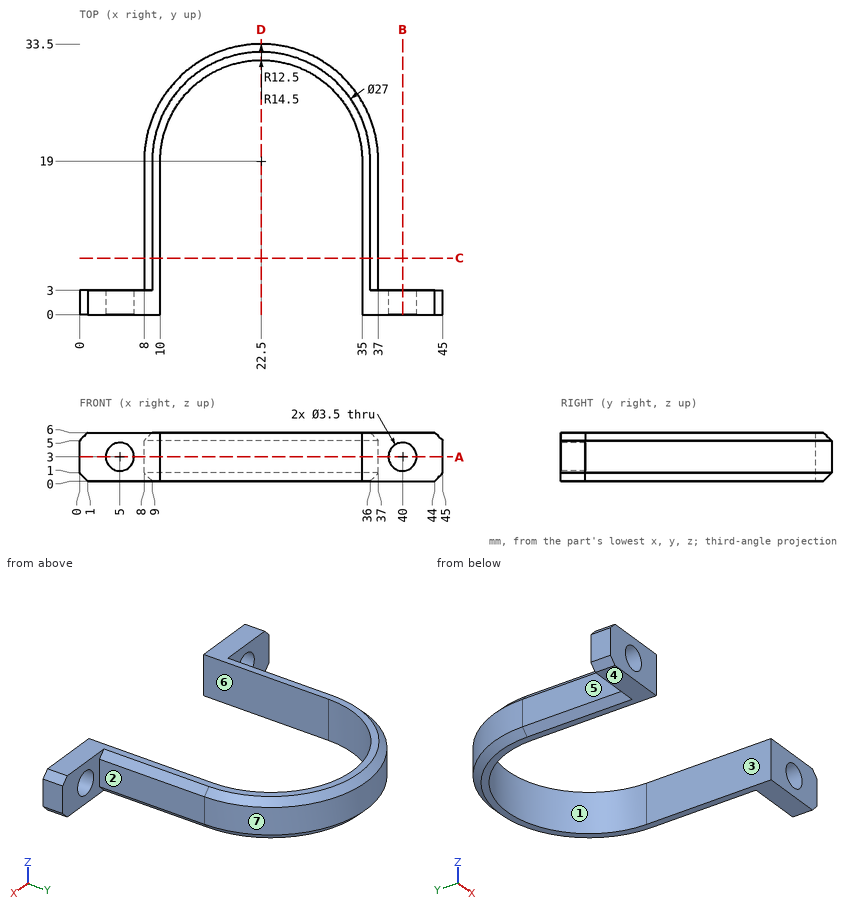
Answer from the drawing. Dimensions are ordinates in mm from the lowest x, y and z of the part. A direction names the side the tool comes from. Round coordinates to 2 decimals unless told otherwise and drop trailing zeros. Loops run counter-clockwise (first coordinate to the right, second up) from the corner with the lowest first, then second, coordinate; pieces in that order, holes last.
1) A cutting plane is placed at D-D on x = 22.5. Determine the outline of the cut face in (y, z).
Outcome:
outline: (31.5, 0) - (32.5, 0) - (33.5, 1) - (33.5, 5) - (32.5, 6) - (31.5, 6) - close
2) Consider line 1 (X direction, y = 16, z = 3.5); line 2 (Z direction, x = 5, y = 1.3); line 3 (X direction, y = 2.5, z = 4). Determine where each line is inside the solid, lowest interval first.
Outcome:
line 1: x = 8 to 10, 35 to 37
line 2: z = 0 to 1.25, 4.75 to 6
line 3: x = 0 to 3.56, 6.44 to 10, 35 to 38.56, 41.44 to 45
3) A cutting plane is placed at B-B on x = 40. Determine the outline of the cut face in (y, z), plus the area to 3 significant figures.
Outcome:
outline: (0, 0) - (3, 0) - (3, 1.25) - (0, 1.25) - close; (0, 4.75) - (3, 4.75) - (3, 6) - (0, 6) - close
area: 7.50 mm2
4) For the marked faces 5, 6 and 7, determine the directions among +Z, -Z, +X, -X, +Y, -Y from which every point of the face is accessible in a straight line to the end or side of a thin tool.
Outcome:
face 5: +Z, -Z, -X, +Y
face 6: +Z, -Z, -Y
face 7: +Z, -Z, +Y
5) A cutting plane is placed at C-C on y = 7. Determine the outline of the cut face in (x, z), plus the area to 3 significant figures.
Outcome:
outline: (8, 1) - (9, 0) - (10, 0) - (10, 6) - (9, 6) - (8, 5) - close; (35, 0) - (36, 0) - (37, 1) - (37, 5) - (36, 6) - (35, 6) - close
area: 22.0 mm2
6) For a pull along X with two mould halves and no side action, classify the marked faces 1, 2, 3 and 4 as released by +X, released by -X, zero draft, split by the parting line, or undercut.
Outcome:
face 1: undercut
face 2: released by +X
face 3: undercut
face 4: zero draft
7) Given P1, Ø2, axis at y = 15.5, z = 4.5, coming from the -X side; P2, Ø2, axis at y = 24.5, z = 4, coming from the +X side; P3, Ø3, axis at y = 8.5, z = 3, coming from the +X side; P4, Ø3, axis at x = 40, z = 3, coming from the -Y side, each flat-ended and moving along its own axis, determine where each tip first touches the part or whether it passes through.
Outcome:
P1: stops at x = 8
P2: stops at x = 36.28
P3: stops at x = 37
P4: passes through
8) A cutting plane is placed at A-A on z = 3. Determine the outline of the cut face in (x, y), plus the area to 3 significant figures.
Outcome:
outline: (0, 0) - (3.25, 0) - (3.25, 3) - (0, 3) - close; (6.75, 0) - (10, 0) - (10, 19) arc R12.5 cw to (35, 19) - (35, 0) - (38.25, 0) - (38.25, 3) - (37, 3) - (37, 19) arc R14.5 ccw to (8, 19) - (8, 3) - (6.75, 3) - close; (41.75, 0) - (45, 0) - (45, 3) - (41.75, 3) - close
area: 188 mm2
